from build123d import *

# Parameters (mm, degrees)
F1_DEPTH = 120


with BuildPart() as f1:
    # F0 (on Front) → F1 (new body)
    with BuildSketch(Plane.XZ):
        Polygon((356.159233, 498.875577), (356.159233, 518.875577), (-343.840767, 518.875577), (-343.840767, 498.875577), (-315.556496, 498.875577), (-165.556496, 498.875577), (-145.556496, 498.875577), align=None)
        Polygon((-315.556496, 498.875577), (-343.840767, 498.875577), (178.866161, -23.83135), (198.866161, -43.83135), (348.866161, -193.83135), (376.951969, -193.83135), (376.951969, -194.545249), (377.40815, -194.089068), (-145.556496, 328.875577), (-165.556496, 348.875577), align=None)
        Polygon((-145.556496, 328.875577), (-145.556496, 498.875577), (-165.556496, 498.875577), (-165.556496, 348.875577), align=None)
        Polygon((198.866161, -43.83135), (178.866161, -23.83135), (178.866161, -193.83135), (198.866161, -193.83135), align=None)
        Polygon((198.866161, -193.83135), (178.866161, -193.83135), (-343.840767, -193.83135), (-343.840767, -213.83135), (376.951969, -213.83135), (376.951969, -194.545249), (376.951969, -193.83135), (348.866161, -193.83135), align=None)
    extrude(amount=F1_DEPTH)


solid = f1.part
Could you check a few things on this model? Use its own coordinates, in mm. A direction names the side the tool comes from. Give positions to 0.01 mm unless a question says otherwise; leave off trailing zeros. Write each loop counter-clockwise with the first axis right and the second up, starting at its lowest first coordinate (ties: lowest second). Pieces come first, ordered by that corner, then holes. Notation, with made-up numbers: (69, 55) -> (121, 55) arc R32 ccw to (121, 91) -> close; hole circle Ø11 at (-15, 66). An arc over 180 degrees is marked (long way). Answer as CSV lines item,"result". Start each with the question number.
(1) If we section it at D-D, the plane z = 288.5: Write out the boundary of the cut face in (x, y).
(2) Please list where these lines run through material, in increasing order: line 1 (Z direction, x = -220, y = -45.5); line 2 (Z direction, x = -207, y = -57); line 3 (X direction, y = -103.5, z = -52.5).
(3) If we section it at A-A, the plane x = -277: Write out the boundary of the cut face in (y, z), and give its area (3 significant figures).
(4) Which directions (+Z, -Z, +X, -X, +Y, -Y) give clear straight access to the entire face, cutting with the end or side of a thin tool? Please do faces 1 (the face through (-79, -59, -193.831)), 2 (the face through (272.816, -59.16, -117.781)), 3 (the face through (-145.556, -59, 413)).
(5) I'm going to push flat-ended pins straight in: pin 1 Ø22 at (y, z) = (-77.5, 504.5) entering from +X; pin 2 Ø5 at (y, z) = (-53.5, 267.5) entering from -X; pin 3 Ø1.5 at (y, z) = (-85.5, 158) entering from +X. Where does each tip first touch, or does it pass through?
(6) If we section it at C-C, the plane y = -15.5: Write out the boundary of the cut face in (x, z).
(7) If we section it at B-B, the plane z = -64.5: Write out the boundary of the cut face in (x, y).
(8) If we mould it in two halves opening along X, with no side actions, what happens to faces 4 (the face through (376.952, -59, -204)), 5 (the face through (11, -59, 518.876)), 6 (the face through (-165.556, -59, 425))? For each: +X half, -X half, draft (parallel to the pull), parting line (faces both ways), or undercut.
Answer list:
1,outline,"(-133.47, -120) -> (-105.18, -120) -> (-105.18, 0) -> (-133.47, 0) -> close"
2,line 1,"-213.83 to -193.83, 375.03 to 403.32, 498.88 to 518.88"
2,line 2,"-213.83 to -193.83, 362.03 to 390.32, 498.88 to 518.88"
2,line 3,"178.87 to 198.87, 207.53 to 235.82"
3,outline,"(-120, -213.83) -> (0, -213.83) -> (0, -193.83) -> (-120, -193.83) -> close; (-120, 432.03) -> (0, 432.03) -> (0, 460.32) -> (-120, 460.32) -> close; (-120, 498.88) -> (0, 498.88) -> (0, 518.88) -> (-120, 518.88) -> close"
3,area,"8,190 mm^2"
4,face 1,"-X, +Y, -Y"
4,face 2,"+Y, -Y"
4,face 3,"+X, +Y, -Y"
5,pin 1,"x = 356.16"
5,pin 2,"x = -114.97"
5,pin 3,"x = 26.07"
6,outline,"(-343.84, -213.83) -> (376.95, -213.83) -> (376.95, -194.55) -> (377.41, -194.09) -> (-145.56, 328.88) -> (-145.56, 498.88) -> (356.16, 498.88) -> (356.16, 518.88) -> (-343.84, 518.88) -> (-343.84, 498.88) -> (178.87, -23.83) -> (178.87, -193.83) -> (-343.84, -193.83) -> close; hole (-315.56, 498.88) -> (-165.56, 348.88) -> (-165.56, 498.88) -> close; hole (198.87, -193.83) -> (348.87, -193.83) -> (198.87, -43.83) -> close"
7,outline,"(178.87, -120) -> (198.87, -120) -> (198.87, 0) -> (178.87, 0) -> close; (219.53, -120) -> (247.82, -120) -> (247.82, 0) -> (219.53, 0) -> close"
8,face 4,"+X half"
8,face 5,"draft"
8,face 6,"undercut"
